The model under review builds one solid part; all positions refer to its coordinate system, in mm. A direction names the side the tool comes from. Coordinates: 2 decimals unless noted, no trailing zeros. Loops run counter-clockwise (first coordinate to the right, second up) from the corner with the lowest first, then second, coordinate; pieces in that order, holes last. Notation, with made-up numbers: (63.25, -12) - (115.25, -12) arc R28 cw to (115.25, 21) - close; hole circle Ø2 at (65.5, 30.25). An arc over 180 degrees is marked (long way). Answer in a Markdown table with one row per item. Add a question column.
(1) For P1, Ø12, axis at x = 24, z = -22, coming from the +Y side; P2, Ø3, axis at y = 0, z = 26.5, coming from the +X side; P3, Ø8, axis at x = -20.5, y = 6, coming from the -Z side; P4, Ø20, axis at x = 13, z = -14.5, coming from the +Y side, all flat-tipped, find the tip position at first contact; note any pin that passes through.
(2) We need section A-A on x = 0. Write out the cut boundary in (y, z), plus the area to 3 significant figures.
(3) We need section C-C on y = 0.75. Write out the cut boundary in (x, z).
(4) For line 1 along X through (y, z) = (3, 0); line 2 along Z through (x, y) = (-29.5, 1.5); line 3 along X through (y, z) = (4.5, 14.5), list the stretches that pass through material, from the lowest coordinate up.
(5) Machinability: for faces 5 (the cylindrical face through (-32.703, 3.415, -7.262)), 6 (the flat face through (28, -8.5, -18)), which of the approach directions +Z, -Z, +X, -X, +Y, -Y give a long, thin tool a straight path to every point of the face, cutting with its end or side? Answer none if there is none.
(6) We need section B-B on z = 0. Write out the cut boundary in (x, y).
(7) Mouldability with a two-part tool opening along X and no side actions: class faces 1 (the conical face through (-30.674, -3.183, -6.812)), 2 (the flat face through (-30.5, 8.5, 15.5)), 3 (the cylindrical face through (23.62, 0.14, -25.76)), 4 (the flat face through (27.5, -1.3, 17.5)) as +X half, -X half, draft (parallel to the pull), parting line (faces both ways), or undercut.
from build123d import *


with BuildPart() as f1:
    # F0 (on Right) → F1 (revolve)
    with BuildSketch(Plane.YZ):
        with BuildLine():
            Line((8, 34.95), (-7.5, 34.95))
            ThreePointArc((-7.5, 34.95), (-8.207107, 34.657107), (-8.5, 33.95))
            Line((-8.5, 33.95), (-8.5, 32.648965))
            ThreePointArc((-8.5, 32.648965), (-8.225374, 31.96061), (-7.552336, 31.650335))
            Line((-7.552336, 31.650335), (-2.352336, 31.377815))
            ThreePointArc((-2.352336, 31.377815), (-1.611645, 31.65107), (-1.3, 32.376444))
            Line((-1.3, 32.376444), (-1.3, 33.5))
            Line((-1.3, 33.5), (8, 33.5))
            ThreePointArc((8, 33.5), (8.353553, 33.646447), (8.5, 34))
            Line((8.5, 34), (8.5, 34.45))
            ThreePointArc((8.5, 34.45), (8.353553, 34.803553), (8, 34.95))
        make_face()
    revolve(axis=Axis((0, -1.514213, 0), (0, 1, 0)))


solid = f1.part
Outcome:
| question | item | result |
|---|---|---|
| 1 | P1 | y = 8.5 |
| 1 | P2 | x = 24.42 |
| 1 | P3 | z = -30.81 |
| 1 | P4 | through |
| 2 | outline | (-8.5, -33.95) arc R1 ccw to (-7.5, -34.95) - (8, -34.95) arc R0.5 ccw to (8.5, -34.45) - (8.5, -34) arc R0.5 ccw to (8, -33.5) - (-1.3, -33.5) - (-1.3, -32.38) arc R1 ccw to (-2.35, -31.38) - (-7.55, -31.65) arc R1 ccw to (-8.5, -32.65) - close; (-8.5, 32.65) arc R1 ccw to (-7.55, 31.65) - (-2.35, 31.38) arc R1 ccw to (-1.3, 32.38) - (-1.3, 33.5) - (8, 33.5) arc R0.5 ccw to (8.5, 34) - (8.5, 34.45) arc R0.5 ccw to (8, 34.95) - (-7.5, 34.95) arc R1 ccw to (-8.5, 33.95) - close |
| 2 | area | 76.4 mm² |
| 3 | outline | circle Ø69.9 at (0, 0); hole circle Ø67 at (0, 0) |
| 4 | line 1 | -34.95 to -33.5, 33.5 to 34.95 |
| 4 | line 2 | -18.74 to -15.87, 15.87 to 18.74 |
| 4 | line 3 | -31.8 to -30.2, 30.2 to 31.8 |
| 5 | face 5 | +Y |
| 5 | face 6 | +Z, -Z, +X, -X, -Y |
| 6 | outline | (-34.95, -7.5) arc R1 ccw to (-33.95, -8.5) - (-32.65, -8.5) arc R1 ccw to (-31.65, -7.55) - (-31.38, -2.35) arc R1 ccw to (-32.38, -1.3) - (-33.5, -1.3) - (-33.5, 8) arc R0.5 ccw to (-34, 8.5) - (-34.45, 8.5) arc R0.5 ccw to (-34.95, 8) - close; (31.38, -2.35) - (31.65, -7.55) arc R1 ccw to (32.65, -8.5) - (33.95, -8.5) arc R1 ccw to (34.95, -7.5) - (34.95, 8) arc R0.5 ccw to (34.45, 8.5) - (34, 8.5) arc R0.5 ccw to (33.5, 8) - (33.5, -1.3) - (32.38, -1.3) arc R1 ccw to start |
| 7 | face 1 | undercut |
| 7 | face 2 | draft |
| 7 | face 3 | parting line |
| 7 | face 4 | undercut |
